The listing builds one solid part. Answer for the finished solid, in the listing's coordinates (mm). A direction names the side the tool comes from. Give positions to 0.01 mm unless a question says otherwise; leave off trailing zeros. Write each loop counter-clockwise with the first axis right and the second up, starting at its lowest first coordinate (ties: lowest second). Pieces come first, ordered by that corner, then holes. Notation, with made-up numbers: (82.5, 31) -> (129.5, 31) arc R24 cw to (129.5, 47) -> close; hole circle Ø5 at (50, 5.5). An arc over 180 degrees is marked (long way). Use CSV: the item, a comma, the result in double quotes. Start each with the question number.
from build123d import *

# Parameters (mm, degrees)
BOSS_EXTRUDE1_DEPTH      = 490.140625
BOSS_EXTRUDE1_DEPTH_BACK = 490.140625
SKETCH3_R                = 24.13
SKETCH6_OUTSIDE_W        = 776.952
SKETCH6_OUTSIDE_H        = 776.952
SKETCH6_OUTSIDE_R        = 22.540972993
CUT_EXTRUDE2_DEPTH       = 986.634670258
CUT_EXTRUDE2_DRAFT       = -15
SKETCH7_OUTSIDE_W        = 776.952
SKETCH7_OUTSIDE_H        = 776.952
SKETCH7_OUTSIDE_R        = 22.540972993
CUT_EXTRUDE3_DEPTH       = 986.634670258
CUT_EXTRUDE3_DRAFT       = -15
BOSS_EXTRUDE2_DEPTH      = 511.175
BOSS_EXTRUDE2_DEPTH_BACK = 511.175


with BuildPart() as part:
    # Sketch2 → Revolve1 (revolve)
    with BuildSketch(Plane.XY, mode=Mode.PRIVATE) as revolve1_sk:
        Polygon((-493.7125, 0), (-493.7125, 11.1125), (-491.33125, 11.1125), (-491.33125, 22.540972993), (-490.140625, 22.86), (-490.140625, 0), align=None)
    revolve(revolve1_sk.sketch.rotate(Axis((-493.7125, 0, 0), (1, 0, 0)), 180), axis=Axis((-493.7125, 0, 0), (1, 0, 0)))


with BuildPart() as body_2:
    # Mirror2: mirrored copy
    add(part.part.mirror(Plane(origin=(0, 0, 0), x_dir=(0, 0, 1), z_dir=(1, 0, 0))))


with BuildPart() as body_3:
    # Sketch3 → Boss-Extrude1 (new, two sides: drawn at the far end of the back side and taken through both)
    with BuildSketch(Plane(origin=(0, 0, 0), x_dir=(0, 0, -1), z_dir=(1, 0, 0)).offset(-BOSS_EXTRUDE1_DEPTH_BACK)):
        Circle(SKETCH3_R)
    extrude(amount=BOSS_EXTRUDE1_DEPTH + BOSS_EXTRUDE1_DEPTH_BACK)


with BuildPart() as cut_extrude2_tool:
    # Sketch6 outside → Cut-Extrude2 (with draft: the straight prism first)
    with BuildSketch(Plane.ZY.offset(491.33125)):
        Rectangle(SKETCH6_OUTSIDE_W, SKETCH6_OUTSIDE_H)
        Circle(SKETCH6_OUTSIDE_R, mode=Mode.SUBTRACT)
    extrude(amount=-CUT_EXTRUDE2_DEPTH)
    # Cut-Extrude2: the draft: its side faces are tilted about the plane it starts from
    cut_extrude2_sides = [cut_extrude2_tool.faces().sort_by_distance(p)[0] for p in [
        (1.986085129, -388.476, 0),
        (1.986085129, 0, 388.476),
        (1.986085129, 388.476, 0),
        (1.986085129, 0, -388.476),
        (1.986085129, 0, -22.540972993),
    ]]
    draft(cut_extrude2_sides, Plane.ZY.offset(491.33125), CUT_EXTRUDE2_DRAFT)


with BuildPart() as body_3_1:
    add(body_3.part)

    # Cut-Extrude2: cut by cut_extrude2_tool
    add(cut_extrude2_tool.part, mode=Mode.SUBTRACT)


with BuildPart() as cut_extrude3_tool:
    # Sketch7 outside → Cut-Extrude3 (with draft: the straight prism first)
    with BuildSketch(Plane(origin=(491.33125, 0, 0), x_dir=(0, 0, -1), z_dir=(1, 0, 0))):
        Rectangle(SKETCH7_OUTSIDE_W, SKETCH7_OUTSIDE_H)
        Circle(SKETCH7_OUTSIDE_R, mode=Mode.SUBTRACT)
    extrude(amount=-CUT_EXTRUDE3_DEPTH)
    # Cut-Extrude3: the draft: its side faces are tilted about the plane it starts from
    cut_extrude3_sides = [cut_extrude3_tool.faces().sort_by_distance(p)[0] for p in [
        (-1.986085129, -388.476, 0),
        (-1.986085129, 0, -388.476),
        (-1.986085129, 388.476, 0),
        (-1.986085129, 0, 388.476),
        (-1.986085129, 0, 22.540972993),
    ]]
    draft(cut_extrude3_sides, Plane(origin=(491.33125, 0, 0), x_dir=(0, 0, -1), z_dir=(1, 0, 0)), CUT_EXTRUDE3_DRAFT)


with BuildPart() as body_3_2:
    add(body_3_1.part)

    # Cut-Extrude3: cut by cut_extrude3_tool
    add(cut_extrude3_tool.part, mode=Mode.SUBTRACT)


with BuildPart() as part_1:
    add(part.part)

    add(body_2.part)  # Boss-Extrude2 merges body 2

    add(body_3_2.part)  # Boss-Extrude2 merges body 3
    # Sketch4 → Boss-Extrude2 (add, two sides: drawn at the far end of the back side and taken through both)
    with BuildSketch(Plane(origin=(0, 0, 0), x_dir=(0, 0, -1), z_dir=(1, 0, 0)).offset(-BOSS_EXTRUDE2_DEPTH_BACK)):
        Polygon((0, 6.415804866), (-5.55625, 3.207902433), (-5.55625, -3.207902433), (0, -6.415804866), (5.55625, -3.207902433), (5.55625, 3.207902433), align=None)
    extrude(amount=BOSS_EXTRUDE2_DEPTH + BOSS_EXTRUDE2_DEPTH_BACK)

    # Sketch5 → Cut-Revolve1 (revolve, cut)
    with BuildSketch(Plane.XY, mode=Mode.PRIVATE) as cut_revolve1_sk:
        with BuildLine():
            Line((-428.30115, 24.1554), (-428.30115, 24.7904))
            Line((-428.30115, 24.7904), (-421.96385, 24.7904))
            Line((-421.96385, 24.7904), (-421.96385, 24.1554))
            ThreePointArc((-421.96385, 24.1554), (-422.52062588, 23.92477588), (-422.75125, 23.368))
            ThreePointArc((-422.75125, 23.368), (-425.1325, 20.98675), (-427.51375, 23.368))
            ThreePointArc((-427.51375, 23.368), (-427.74437412, 23.92477588), (-428.30115, 24.1554))
        make_face()
    revolve(cut_revolve1_sk.sketch.rotate(Axis((-511.175, 0, 0), (1, 0, 0)), 180), axis=Axis((-511.175, 0, 0), (1, 0, 0)), mode=Mode.SUBTRACT)


solid = part_1.part
Q1. Section A-A on x = -23.5 is taken. Give the vertices of the cut face in (y, z), then the cut area to 3 significant figures.
Q2. Straight lines are drawn through the part: L1, parallel to Y at x = 201.5, z = 9; L2, parallel to X at y = -1, z = 10; L3, parallel to X at y = 22, z = 0.5. For each, find the intervals that lie inside material, in ascending order.
Q3. Flat-ended cylindrical pins translate along their axes: pin 1 Ø1.5 at (x, z) = (256.5, -16) entering from -Y; pin 2 Ø12 at (x, y) = (-98, -13) entering from +Z; pin 3 Ø1.9 at (x, y) = (-499, 1) entering from +Z; pin 4 Ø6 at (x, z) = (13.5, -0.5) entering from -Y. Find the tip coordinate at first contact, or state that the pin passes through.
Q4. For faces 1 (the face through (25.266, 7.248, -23.016)), 2 (the face through (-493.712, -5, -3)), 3 (the face through (493.712, -5, -3)), determine the directions among +Z, -Z, +X, -X, +Y, -Y from which every point of the face is accessible in a straight line to the end or side of a thin tool.
Output:
1,outline,"circle Ø48.26 at (0, 0)"
1,area,"1,830 mm²"
2,L1,"-22.39 to 22.39"
2,L2,"-493.71 to 493.71"
2,L3,"-491.33 to -427.09, -423.18 to 491.33"
3,pin 1,"y = -18.7"
3,pin 2,"z = 23.09"
3,pin 3,"z = 5.56"
3,pin 4,"y = -24.13"
4,face 1,"+X, -X"
4,face 2,"-X"
4,face 3,"+X"
